Here's how the part is built. I have some questions about the finished solid (model axes, mm). A direction names the side the tool comes from. Coordinates: 2 decimals unless noted, no trailing zeros. Loops run counter-clockwise (first coordinate to the right, second up) from the corner with the lowest first, then second, coordinate; pieces in that order, holes last. Notation, with made-up numbers: M 42.5,58 L 92.5,58 A14 cw 92.5,71 Z; hole C 32,84.25 d8. An arc over 180 degrees is marked long. Use one line per item in the form item = value. Start each with the question number.
(1) Thinking about a two-plate mould opening in Z: for faces 4 (the flat face through (-38.1, 0, 0)), 5 (the cylindrical face through (34.836, 0.462, 34.796)), 6 (the cylindrical face through (36.651, 0.462, 36.572)), 7 (the cylindrical face through (0.462, -34.836, 34.796)), which applies, +Z half, -Z half, draft (parallel to the pull), parting line (faces both ways), or undercut?
(2) Will these pins go through, and if not, where does the flat tip stop? P1, Ø1.3, axis at y = -2.5, z = 37, coming from the -X side; P2, Ø3, axis at x = 11, z = 37, coming from the -Y side; P3, Ø6, axis at x = 13.5, y = 12, coming from the +Z side.
(3) Please list where these lines run through material, in increasing order: L1, parallel to X at y = -11, z = -25.5; L2, parallel to Z at x = 27.5, y = -28.5.
(4) Imagine slicing it at A-A, the plane z = -2.5. Please give me the cut outline in (x, y).
(5) On a 3-axis mill with a long thin cutter (end or side, diameter ignored), from which of +Z, -Z, +X, -X, +Y, -Y can I reach the whole of each face in a straight line? I mean faces 1 (the cylindrical face through (0.462, -36.651, 36.572)), 2 (the flat face through (0, 0, -35.56)), 3 (the cylindrical face through (0.462, 34.796, 34.836)). Say none if no direction works.
(6) Imagine slicing it at B-B, the plane y = 15. Please give me the cut outline in (x, z), and give its area (3 significant figures).
```python
from build123d import *

# Parameters (mm, degrees)
F0_W     = 76.2
F0_H     = 76.2
F1_DEPTH = 38.1
F2_R     = 5.08
F3_T     = -2.54


# Not quite as in the source:
# - a shell that OpenCascade refuses in one call is made with other operations: the cavity is built on its own and cut out


with BuildPart() as f1:
    # F0 (on Front) → F1 (new body, symmetric)
    with BuildSketch(Plane.XZ):
        Rectangle(F0_W, F0_H)
    extrude(amount=F1_DEPTH, both=True)

    # F2
    f2_edges = [f1.edges().sort_by_distance(p)[0] for p in [
        (0, 38.1, 38.1),
        (-38.1, 0, 38.1),
        (0, -38.1, 38.1),
        (38.1, 0, 38.1),
        (38.1, 38.1, 0),
        (38.1, -38.1, 0),
        (38.1, 0, -38.1),
        (-38.1, -38.1, 0),
        (0, -38.1, -38.1),
        (-38.1, 0, -38.1),
        (0, 38.1, -38.1),
        (-38.1, 38.1, 0),
    ]]
    fillet(f2_edges, radius=F2_R)

    # F3: a shell. OpenCascade refuses it in one call, so the cavity is built on its own and cut out:
    # the body offset inwards by the wall thickness, plus a prism from it out through each open face.
    f3_core = offset(f1.part, amount=F3_T, mode=Mode.PRIVATE)
    f3_exits = [f3_core.faces().sort_by_distance(p)[0] for p in [
        (0, 0, 35.56),
    ]]
    add(f3_core, mode=Mode.SUBTRACT)
    extrude(f3_exits, amount=-F3_T, mode=Mode.SUBTRACT)


solid = f1.part
```
Answer:
q1.face_4 = draft
q1.face_5 = undercut
q1.face_6 = +Z half
q1.face_7 = undercut
q2.P1 = -36.86
q2.P2 = -37.45
q2.P3 = -35.56
q3.L1 = -38.1 to -35.56, 35.56 to 38.1
q3.L2 = -38.1 to -35.56
q4.outline = M -38.1,-33.02 A5.08 ccw -33.02,-38.1 L 33.02,-38.1 A5.08 ccw 38.1,-33.02 L 38.1,33.02 A5.08 ccw 33.02,38.1 L -33.02,38.1 A5.08 ccw -38.1,33.02 Z; hole M -35.56,-33.02 A2.54 ccw -33.02,-35.56 L 33.02,-35.56 A2.54 ccw 35.56,-33.02 L 35.56,33.02 A2.54 ccw 33.02,35.56 L -33.02,35.56 A2.54 ccw -35.56,33.02 Z
q5.face_1 = +Z, +X, -X, -Y
q5.face_2 = +Z
q5.face_3 = none
q6.outline = M -38.1,-33.02 A5.08 ccw -33.02,-38.1 L 33.02,-38.1 A5.08 ccw 38.1,-33.02 L 38.1,33.02 A5.08 ccw 33.02,38.1 L 33.02,35.56 A2.54 cw 35.56,33.02 L 35.56,-33.02 A2.54 cw 33.02,-35.56 L -33.02,-35.56 A2.54 cw -35.56,-33.02 L -35.56,33.02 A2.54 cw -33.02,35.56 L -33.02,38.1 A5.08 ccw -38.1,33.02 Z
q6.area = 564 mm²
